from build123d import *

# Parameters (mm, degrees)
F0_W     = 105
F0_H     = 70
F1_DEPTH = 50
F3_DEPTH = 105.001
F5_DEPTH = 105.001
F6_W     = 65
F6_H     = 40
F7_DEPTH = 70.001
F9_DEPTH = 105.001


with BuildPart() as f1:
    # F0 (on Top) → F1 (new body)
    with BuildSketch(Plane.XY):
        Rectangle(F0_W, F0_H)
    extrude(amount=F1_DEPTH)

    # F2 (on face) → F3 (cut, through all)
    with BuildSketch(Plane.YZ.offset(52.5)):
        Polygon((16, 0), (35, 0), (35, 19), align=None)
    extrude(amount=-F3_DEPTH, mode=Mode.SUBTRACT)

    # F4 (on face) → F5 (cut, through all)
    with BuildSketch(Plane.YZ.offset(52.5)):
        Polygon((-44.933475, 79.933475), (-35, 20), (15, 20), align=None)
    extrude(amount=-F5_DEPTH, mode=Mode.SUBTRACT)

    # F6 (on face) → F7 (cut, through all)
    with BuildSketch(Plane.XZ.offset(35)):
        Rectangle(F6_W, F6_H)
    extrude(amount=-F7_DEPTH, mode=Mode.SUBTRACT)

    # F8 (on face) → F9 (cut, through all)
    with BuildSketch(Plane(origin=(-52.5, 0, 0), x_dir=(0, -1, 0), z_dir=(-1, 0, 0))):
        Polygon((35, 0), (35, 20), (-15, 20), align=None)
    extrude(amount=-F9_DEPTH, mode=Mode.SUBTRACT)


solid = f1.part
Verification items for the finished model (mm, model axes). A direction names the side the tool comes from. Coordinates: 2 decimals unless noted, no trailing zeros. Order: outer loops, then holes, each group sorted by start corner. A loop starts at its lowest first (then second) coordinate and runs counter-clockwise, first axis right, second up. Notation, with made-up numbers: M 76,-35 L 103,-35 A23 ccw 103,-9 Z; hole C 55,26 d11. An arc over 180 degrees is marked long. Return JSON: item names as keys, results as strings.
1) Cross-section at A-A, the plane y = -29.5. Record the boundary of the cut face in (x, z).
Answer list:
{"outline": "M -52.5,0 L -32.5,0 L -32.5,2.2 L -52.5,2.2 Z; M 32.5,0 L 52.5,0 L 52.5,2.2 L 32.5,2.2 Z"}
2) Release check for a two-part mould opening along X. For faces 1 (the flat face through (52.5, 15, 25)), 2 (the flat face through (42, -9, 0)), 3 (the flat face through (32.5, 7, 8)) record: +X half, -X half, draft (parallel to the pull), parting line (faces both ways), or undercut.
Answer list:
{"face 1": "+X half", "face 2": "draft", "face 3": "undercut"}
3) Cross-section at B-B, the plane z = 7.5. Record the boundary of the cut face in (x, y), and give its area (3 significant figures).
Answer list:
{"outline": "M -52.5,-16.25 L -32.5,-16.25 L -32.5,23.5 L -52.5,23.5 Z; M 32.5,-16.25 L 52.5,-16.25 L 52.5,23.5 L 32.5,23.5 Z", "area": "1,590 mm2"}
4) Cross-section at C-C, the plane y = -10. Record the boundary of the cut face in (x, z), and give its area (3 significant figures).
Answer list:
{"outline": "M -52.5,0 L -32.5,0 L -32.5,10 L -52.5,10 Z; M -52.5,45 L 52.5,45 L 52.5,50 L -52.5,50 Z; M 32.5,0 L 52.5,0 L 52.5,10 L 32.5,10 Z", "area": "925 mm2"}
5) Thickness scan on L1, parallel to X at y = -0.5, z = 11; L2, parallel to Z at x = 43, y = 11; L3, parallel to Z at x = 4.5, y = 17.5. Record the ranges inside material, lowest first. Write a range as [from, to].
Answer list:
{"L1": "[-52.5, -32.5], [32.5, 52.5]", "L2": "[0, 18.4], [24, 50]", "L3": "[20, 50]"}
6) Cross-section at D-D, the plane y = 29. Record the boundary of the cut face in (x, z).
Answer list:
{"outline": "M -52.5,13 L -32.5,13 L -32.5,20 L 32.5,20 L 32.5,13 L 52.5,13 L 52.5,50 L -52.5,50 Z"}
7) Gauge pin test, flat ends, axial feed: pin 1 (6 mm diameter, centred on x = 19.5, z = 22.5, fed in from -Y); pin 2 (8 mm diameter, centred on x = -19, y = -1, fed in from -Z); pin 3 (16 mm diameter, centred on x = -8.5, y = 29.5, fed in from -Z). Record the tip position at first contact, or that the pin passes through.
Answer list:
{"pin 1": "y = 9.5", "pin 2": "z = 32", "pin 3": "z = 20"}
8) Access from +Z, -Z, +X, -X, +Y, -Y to the whole of each face (thin tool, end or side, straight path). Record for faces 4 (the flat face through (-42, 26, 10)), 5 (the flat face through (-43, -10, 10)), 6 (the flat face through (-32.5, 7, 8)).
Answer list:
{"face 4": "-Z, +X, -X, +Y", "face 5": "+X, -X, -Y", "face 6": "-Z, +Y, -Y"}
